Input: part model. Units: mm. Frame: model coordinates. A direction names the side the tool comes from. Round coordinates to 2 decimals unless told otherwise and drop trailing zeros. Write each loop counter-clockwise with the first axis right and the second up, starting at its lowest first coordinate (ties: lowest second). Pieces come first, ordered by that corner, then holes. Notation, with made-up numbers: (62, 36.5) -> (108, 36.5) arc R25 cw to (108, 49.5) -> close; hole circle Ø7 at (32.5, -0.75). An arc over 180 degrees is marked (long way). Write item = value, one per line.
```python
from build123d import *

# Parameters (mm, degrees)
BASPROSKE_W      = 10
BASPROSKE_H      = 22
TOOTHCUT_DEPTH   = 33.680269277
TEETHCUTS_COUNT  = 20
TEETHCUTS_ANGLE  = 342
HUBNEAONESKE_R   = 15
HUBNEARONE_DEPTH = 15.0000508
BORSKE_R         = 7
BORE_DEPTH       = 25.0000508
CHAMFER_1_SIZE   = 2


with BuildPart() as part:
    # BasProSke → Base-Revolve (revolve)
    with BuildSketch(Plane(origin=(0, 0, 0), x_dir=(1, 0, 0), z_dir=(0, 1, 0)), mode=Mode.PRIVATE) as base_revolve_sk:
        with Locations((5, 11)):
            Rectangle(BASPROSKE_W, BASPROSKE_H)
    revolve(base_revolve_sk.sketch.rotate(Axis((-10, 0, 0), (1, 0, 0)), 180), axis=Axis((-10, 0, 0), (1, 0, 0)))

    # TooCutSke → ToothCut (cut, through all)
    with BuildSketch(Plane(origin=(0, 0, 0), x_dir=(0, 0, -1), z_dir=(1, 0, 0))):
        with BuildLine():
            ThreePointArc((0.986171591, 17.471189616), (0, 17.499), (-0.986171591, 17.471189616))
            ThreePointArc((-0.986171591, 17.471189616), (-1.626916196, 19.798789858), (-2.932850173, 21.829260982))
            ThreePointArc((-2.932850173, 21.829260982), (0, 22.0254), (2.932850173, 21.829260982))
            ThreePointArc((2.932850173, 21.829260982), (1.626916196, 19.798789858), (0.986171591, 17.471189616))
        make_face()
    toothcut = extrude(amount=TOOTHCUT_DEPTH, mode=Mode.SUBTRACT)

    # TeethCuts: ToothCut ×20 about axis
    teethcuts_axis = Axis((-10, 0, 0), (1, 0, 0))
    for i in range(1, TEETHCUTS_COUNT):
        add(toothcut.rotate(teethcuts_axis, i * TEETHCUTS_ANGLE / (TEETHCUTS_COUNT - 1)), mode=Mode.SUBTRACT)

    # HubNeaOneSke → HubNearOne (add)
    with BuildSketch(Plane.ZY):
        with Locations(Location((0, 0, 0), (0, 0, 180))):
            Circle(HUBNEAONESKE_R)
    extrude(amount=HUBNEARONE_DEPTH)

    # BorSke → Bore (cut, symmetric)
    with BuildSketch(Plane(origin=(0, 0, 0), x_dir=(0, 0, -1), z_dir=(1, 0, 0))):
        with Locations(Location((0, 0, 0), (0, 0, 180))):
            Circle(BORSKE_R)
    extrude(amount=BORE_DEPTH, both=True, mode=Mode.SUBTRACT)

    # 倒角1
    chamfer_1_edges = [part.edges().sort_by_distance(p)[0] for p in [
        (-15.0000508, 0, -7),
        (10, 0, -7),
    ]]
    chamfer(chamfer_1_edges, length=CHAMFER_1_SIZE)


solid = part.part
```
1) Cut plane C-C (z = -12). Return the cut outline in (x, y), and give its area (3 significant figures).
Solutions:
outline = (-15, -9) -> (0, -9) -> (0, -14.42) -> (10, -14.42) -> (10, 14.42) -> (0, 14.42) -> (0, 9) -> (-15, 9) -> close
area = 558 mm^2
2) Access query for faces 1 (the face through (4.93, 12.97, 15.07)), 2 (the face through (4.93, -14.17, -10.27)), 3 (the face through (4.93, 1.607, -19.754)), 4 (the face through (4.93, -15.037, -12.911)), 5 (the face through (4.93, 15.037, 12.911)). Directions: +Z, -Z, +X, -X, +Y, -Y. A direction counts if a zero-diameter tool reaches every point of the face in a straight line with its end or side. Return the directions, or none.
Solutions:
face_1 = +Z, +X, -X
face_2 = +X, -X
face_3 = -Z, +X, -X
face_4 = +X, -X, -Y
face_5 = +X, -X, +Y
3) Draft query along Z for faces 6 (the face through (4.93, -12.97, -15.07)), 7 (the face through (5.07, 3.449, 21.728)), 8 (the face through (4.93, 14.17, 10.27)). Return one class per face: +Z half, -Z half, draft (parallel to the pull), parting line (faces both ways), or undercut.
Solutions:
face_6 = -Z half
face_7 = +Z half
face_8 = undercut
4) Line query: L1, parallel to Y at x = -8.5, z = 0; L2, parallel to Y at x = 5.5, z = 15.5; L3, parallel to Z at x = 4.5, y = -2. Output: solid intervals per line, ascending. Write a range as from..to.
Solutions:
L1 = -15..-7, 7..15
L2 = -15.61..-13.84, -9.86..9.86, 13.84..15.61
L3 = -20.53..-6.71, 6.71..20.53
5) Cut plane A-A (z = 0). Return the cut outline in (x, y), and give its area (3 significant figures).
Solutions:
outline = (-15, -15) -> (0, -15) -> (0, -17.5) -> (10, -17.5) -> (10, -9) -> (8, -7) -> (-13, -7) -> (-15, -9) -> close; (-15, 9) -> (-13, 7) -> (8, 7) -> (10, 9) -> (10, 17.5) -> (0, 17.5) -> (0, 15) -> (-15, 15) -> close
area = 442 mm^2
6) Cut plane D-D (x = -6). Return the cut outline in (y, z).
Solutions:
outline = circle Ø30 at (0, 0); hole circle Ø14 at (0, 0)
7) First-contact query: P1, Ø5, axis at y = 17.5, z = 13.5, coming from the -X side; P2, Ø1.5, axis at x = -1, z = -12.5, coming from the +Y side; P3, Ø1.5, axis at x = 3.5, y = 1.5, coming from the +Z side. Flat tips, straight axial feed; report the tip coordinate or a pass-through.
Solutions:
P1 = 0
P2 = 9.32
P3 = 20.94
